```python
from build123d import *

# Parameters (mm, degrees)
SKETCH1_R           = 1.5
SKETCH1_W           = 50
SKETCH1_H           = 22.5
BOSS_EXTRUDE2_DEPTH = 3
SKETCH2_W           = 42
SKETCH2_H           = 30
BOSS_EXTRUDE3_DEPTH = 3
BOSS_EXTRUDE4_START = 39
SKETCH1_2_R         = 1.5
SKETCH1_2_W         = 50
SKETCH1_2_H         = 22.5
BOSS_EXTRUDE4_DEPTH = 3
SKETCH4_W           = 36
SKETCH4_H           = 24
CUT_EXTRUDE1_DEPTH  = 3
SKETCH5_W           = 65
SKETCH5_H           = 42
BOSS_EXTRUDE5_DEPTH = 3
SKETCH6_W           = 65
SKETCH6_H           = 42
BOSS_EXTRUDE6_DEPTH = 3


with BuildPart() as part:
    # Sketch1 → Boss-Extrude2 (new body)
    with BuildSketch(Plane.XY):
        with BuildLine():
            Line((0, 10), (0, 12))
            Line((0, 12), (-10, 12))
            Line((-10, 12), (-10, 15))
            Line((-10, 15), (-81, 15))
            Line((-81, 15), (-81, -15))
            Line((-81, -15), (-10, -15))
            Line((-10, -15), (-10, -12))
            Line((-10, -12), (0, -12))
            Line((0, -12), (0, -10))
            ThreePointArc((0, -10), (10, 0), (0, 10))
        make_face()
        with Locations((0, 7)):
            Circle(SKETCH1_R, mode=Mode.SUBTRACT)
        with Locations((7, 0)):
            Circle(SKETCH1_R, mode=Mode.SUBTRACT)
        with Locations((0, -7)):
            Circle(SKETCH1_R, mode=Mode.SUBTRACT)
        with Locations((-7, 0)):
            Circle(SKETCH1_R, mode=Mode.SUBTRACT)
        with Locations((-20, 11.25)):
            Circle(SKETCH1_R, mode=Mode.SUBTRACT)
        with Locations((-20, -11.25)):
            Circle(SKETCH1_R, mode=Mode.SUBTRACT)
        with Locations((-77.5, 11.25)):
            Circle(SKETCH1_R, mode=Mode.SUBTRACT)
        with Locations((-77.5, -11.25)):
            Circle(SKETCH1_R, mode=Mode.SUBTRACT)
        with Locations((-48.75, 0)):
            Rectangle(SKETCH1_W, SKETCH1_H, mode=Mode.SUBTRACT)
    extrude(amount=BOSS_EXTRUDE2_DEPTH)

    # Sketch2 → Boss-Extrude3 (add)
    with BuildSketch(Plane.ZY.offset(81)):
        with Locations((21, 0)):
            Rectangle(SKETCH2_W, SKETCH2_H)
    extrude(amount=BOSS_EXTRUDE3_DEPTH)

    # Sketch1<2> → Boss-Extrude4 (add)
    with BuildSketch(Plane.XY.offset(BOSS_EXTRUDE4_START)):
        with BuildLine():
            Line((0, 10), (0, 12))
            Line((0, 12), (-10, 12))
            Line((-10, 12), (-10, 15))
            Line((-10, 15), (-81, 15))
            Line((-81, 15), (-81, -15))
            Line((-81, -15), (-10, -15))
            Line((-10, -15), (-10, -12))
            Line((-10, -12), (0, -12))
            Line((0, -12), (0, -10))
            ThreePointArc((0, -10), (10, 0), (0, 10))
        make_face()
        with Locations((0, 7)):
            Circle(SKETCH1_2_R, mode=Mode.SUBTRACT)
        with Locations((7, 0)):
            Circle(SKETCH1_2_R, mode=Mode.SUBTRACT)
        with Locations((0, -7)):
            Circle(SKETCH1_2_R, mode=Mode.SUBTRACT)
        with Locations((-7, 0)):
            Circle(SKETCH1_2_R, mode=Mode.SUBTRACT)
        with Locations((-20, 11.25)):
            Circle(SKETCH1_2_R, mode=Mode.SUBTRACT)
        with Locations((-20, -11.25)):
            Circle(SKETCH1_2_R, mode=Mode.SUBTRACT)
        with Locations((-77.5, 11.25)):
            Circle(SKETCH1_2_R, mode=Mode.SUBTRACT)
        with Locations((-77.5, -11.25)):
            Circle(SKETCH1_2_R, mode=Mode.SUBTRACT)
        with Locations((-48.75, 0)):
            Rectangle(SKETCH1_2_W, SKETCH1_2_H, mode=Mode.SUBTRACT)
    extrude(amount=BOSS_EXTRUDE4_DEPTH)

    # Sketch4 → Cut-Extrude1 (cut)
    with BuildSketch(Plane.ZY.offset(84)):
        with Locations((21, 0)):
            Rectangle(SKETCH4_W, SKETCH4_H)
    extrude(amount=-CUT_EXTRUDE1_DEPTH, mode=Mode.SUBTRACT)

    # Sketch5 → Boss-Extrude5 (add)
    with BuildSketch(Plane(origin=(0, 15, 0), x_dir=(1, 0, 0), z_dir=(0, 1, 0))):
        with Locations((-51.5, -21)):
            Rectangle(SKETCH5_W, SKETCH5_H)
    extrude(amount=BOSS_EXTRUDE5_DEPTH)

    # Sketch6 → Boss-Extrude6 (add)
    with BuildSketch(Plane.XZ.offset(15)):
        with Locations((-51.5, 21)):
            Rectangle(SKETCH6_W, SKETCH6_H)
    extrude(amount=BOSS_EXTRUDE6_DEPTH)


solid = part.part
```
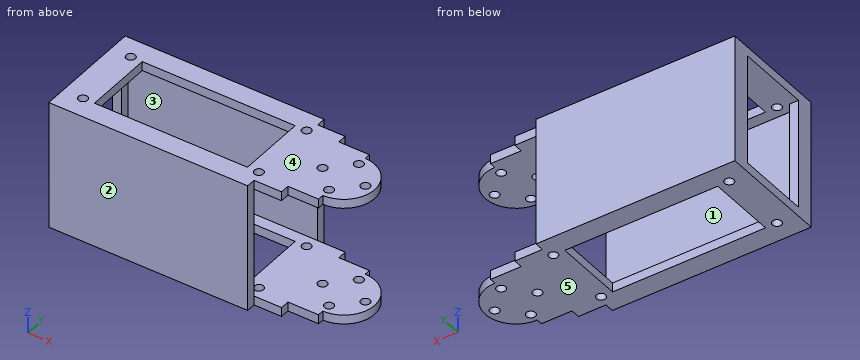
Model file for the job. Use its own axes, mm. Face numbers are marked on the shaded views. A direction names the side the tool comes from. Coordinates: 2 decimals unless noted, no trailing zeros. Write each loop counter-clockwise with the first axis right and the second up, starting at its lowest first coordinate (ties: lowest second). Pieces come first, ordered by that corner, then holes. Notation, with made-up numbers: (1, -14) - (33, -14) arc R21 cw to (33, 16) - close; hole circle Ø9 at (-3.75, 68). An arc over 180 degrees is marked (long way). One line per item, written item: value. Start each with the question number.
1. Slice it at D-D (y = 7). Write the cut outline in (x, z).
2. Slice it at B-B (z = 21.5). Write the cut outline in (x, y), plus the area to 3 significant figures.
3. Mould opens along Z. For the marked faces 3, 4 and 5 say: released by +Z, released by -Z, zero draft, split by the parting line, or undercut.
4. Probe line 1 (Y direction, x = -77.5, z = 40.4); line 2 (Z direction, x = -11, y = -0.5); line 3 (Y direction, x = -63, z = 13). List the from-to ranges inside material, lowest first. Write a range as from..to.
5. Tool access for the marked faces 1 and 2: list every direction of +Z, -Z, +X, -X, +Y, -Y with a clear straight run to the whole face (end or side of a thin tool).
6. Slice it at A-A (x = -20). Write the cut outline in (y, z), plus the area to 3 significant figures.
7. Slice it at C-C (y = 0). Count the separate pieces of the cut face and the enclosed holes in it, plus the area to 3 significant figures.
8. Flat gauge pins, fed straight in: pin 1 (8 mm diameter, centred on y = 4.5, z = 18, fed in from +X); pin 2 (4 mm diameter, centred on x = 7, y = 0, fed in from +Z); pin 3 (1.6 mm diameter, centred on y = 11.5, z = 1.5, fed in from +X); pin 4 (2.5 mm diameter, centred on x = -12.5, z = 1, fed in from -Y). Where does each tip first touch, or does it go through?
Answers below:
1. outline: (-84, 0) - (-73.75, 0) - (-73.75, 3) - (-84, 3) - close; (-84, 39) - (-73.75, 39) - (-73.75, 42) - (-84, 42) - close; (-23.75, 0) - (-1.5, 0) - (-1.5, 3) - (-23.75, 3) - close; (-23.75, 39) - (-1.5, 39) - (-1.5, 42) - (-23.75, 42) - close; (1.5, 0) - (7.14, 0) - (7.14, 3) - (1.5, 3) - close; (1.5, 39) - (7.14, 39) - (7.14, 42) - (1.5, 42) - close
2. outline: (-84, -18) - (-19, -18) - (-19, -15) - (-81, -15) - (-81, -12) - (-84, -12) - close; (-84, 12) - (-81, 12) - (-81, 15) - (-19, 15) - (-19, 18) - (-84, 18) - close
2. area: 408 mm^2
3. face 3: undercut
3. face 4: released by +Z
3. face 5: released by -Z
4. line 1: y = -18..-12.75, -9.75..9.75, 12.75..18
4. line 2: z = 0..3, 39..42
4. line 3: y = -18..-15, 15..18
5. face 1: +X
5. face 2: +Z, -Z, +X, -X, -Y
6. outline: (-18, 0) - (-12.75, 0) - (-12.75, 3) - (-15, 3) - (-15, 39) - (-12.75, 39) - (-12.75, 42) - (-18, 42) - close; (-9.75, 0) - (9.75, 0) - (9.75, 3) - (-9.75, 3) - close; (-9.75, 39) - (9.75, 39) - (9.75, 42) - (-9.75, 42) - close; (12.75, 0) - (18, 0) - (18, 42) - (12.75, 42) - (12.75, 39) - (15, 39) - (15, 3) - (12.75, 3) - close
6. area: 396 mm^2
7. separate pieces: 8
7. enclosed holes: 0
7. area: 228 mm^2
8. pin 1: passes through
8. pin 2: stops at z = 42
8. pin 3: stops at x = 0
8. pin 4: stops at y = -15
